Could you check a few things on this model? Use its own coordinates, in mm. A direction names the side the tool comes from. Round coordinates to 2 decimals unless told otherwise and drop trailing zeros. Write each loop counter-clockwise with the first axis right and the second up, starting at its lowest first coordinate (ties: lowest second). Pieces come first, ordered by that corner, then holes. Notation, with made-up numbers: M 20,42 L 28,42 A11 ccw 28,60 Z; hole C 54.5,69.25 d8. An arc over 180 degrees is marked long. One line per item, written item: value. Start each with the question number.
(1) I want a section at C-C on z = 0.85. Count the separate pieces of the cut face and the enclosed holes in it, and give its area (3 significant figures).
(2) I want a section at B-B on y = 25. Please give me the cut outline in (x, z).
(3) Which directions (+Z, -Z, +X, -X, +Y, -Y) give clear straight access to the entire face, cutting with the end or side of a thin tool? Please do faces 4 (the face through (-35, 50.619, 2)), 5 (the face through (-23, 19.156, 2)), 6 (the face through (-1, 37.156, 2)), 7 (the face through (-14.653, 5, 2)).
(4) I want a section at A-A on x = -29.5. Please give me the cut outline in (y, z), and give its area (3 significant figures).
(5) I'm going to push flat-ended pins straight in: pin 1 Ø2 at (x, z) = (0, 1) entering from -Y; pin 2 Ø2 at (x, z) = (-44.5, 3) entering from -Y; pin 3 Ø3 at (x, y) = (-20.38, 14.02) entering from +Z; pin 4 Ø2 at (x, z) = (-1, 2.5) entering from +Y. Where does each tip first touch, or does it pass through?
(6) If I drill on L1, parallel to X at y = 39.5, z = 3.7; L2, parallel to X at y = 34.5, z = 3.85; L3, parallel to X at y = 44, z = 1.3, over which ranges is the centre line in solid material (lowest first)?
(7) Thinking about a two-plate mould opening in Y: for faces 1 (the face through (-11, 37.156, 2)), 2 (the face through (2.101, 15, 2)), 3 (the face through (0.6, 4.99, 1.97)), which applies, released by +Y, released by -Y, zero draft, split by the parting line, or undercut?
```python
from build123d import *

# Parameters (mm, degrees)
SKETCH1_R           = 1.55
BOSS_EXTRUDE1_DEPTH = 4
SKETCH2_R           = 11.25
CUT_EXTRUDE1_DEPTH  = 10
SKETCH4_R           = 2
SKETCH4_W           = 16.7545444
SKETCH4_H           = 7.593360653
BOSS_EXTRUDE2_DEPTH = 4
SKETCH5_R           = 2.001806379
CUT_EXTRUDE2_DEPTH  = 79.038052705
FILLET1_R           = 5


with BuildPart() as part:
    # Sketch1 → Boss-Extrude1 (new body)
    with BuildSketch(Plane.XY):
        Polygon((-6.898627884, 24.176481231), (-6.898627884, 21.876481231), (-14.898627884, 21.876481231), (-14.898627884, 19.156481231), (-46.856968571, 19.156481231), (-46.856968571, 39.876481231), (-14.898627884, 39.876481231), (-14.898627884, 37.156481231), (-6.898627884, 37.156481231), (-6.898627884, 34.856481231), (-7.878627884, 34.856481231), (-7.878627884, 32.800088029), (-7.031414289, 32.376481231), (-3.77584148, 32.376481231), (-2.928627884, 32.800088029), (-2.928627884, 34.856481231), (-3.898627884, 34.856481231), (-3.898627884, 37.156481231), (2.101372116, 37.156481231), (2.101372116, 47.876481231), (2.101372116, 50.619437371), (-56.558762416, 50.619437371), (-56.558762416, 47.876481231), (-56.558762416, 39.876481231), (-56.558762416, 19.156481231), (-56.558762416, 11.156481231), (2.101372116, 11.156481231), (2.101372116, 21.876481231), (-3.898627884, 21.876481231), (-3.898627884, 24.176481231), (-2.928627884, 24.176481231), (-2.928627884, 26.232874433), (-3.77584148, 26.656481231), (-7.031414289, 26.656481231), (-7.878627884, 26.232874433), (-7.878627884, 24.176481231), align=None)
        with Locations((-51.378627884, 14.016481231)):
            Circle(SKETCH1_R, mode=Mode.SUBTRACT)
        with Locations((-20.378627884, 14.016481231)):
            Circle(SKETCH1_R, mode=Mode.SUBTRACT)
        with Locations((-51.378627884, 45.016481231)):
            Circle(SKETCH1_R, mode=Mode.SUBTRACT)
        with Locations((-20.378627884, 45.016481231)):
            Circle(SKETCH1_R, mode=Mode.SUBTRACT)
    extrude(amount=BOSS_EXTRUDE1_DEPTH)

    # Sketch2 → Cut-Extrude1 (cut)
    with BuildSketch(Plane.XY.offset(4)):
        with Locations((-35.878627884, 29.516481231)):
            Circle(SKETCH2_R)
    extrude(amount=-CUT_EXTRUDE1_DEPTH, mode=Mode.SUBTRACT)

    # Sketch4 → Boss-Extrude2 (add)
    # profile 1 of 2: a face of its own
    with BuildSketch(Plane(origin=(0, 0, 0), x_dir=(-1, 0, 0), z_dir=(0, 0, -1))):
        Polygon((-2.101372116, 50.619437371), (-2.101372116, 53.619437371), (15.109222475, 53.619437371), (15.109222475, 50.619437371), (15.109222475, 46.213030652), (-2.101372116, 46.03430596), align=None)
        with Locations((5.403627884, 49.175308869)):
            Circle(SKETCH4_R, mode=Mode.SUBTRACT)
    # profile 2 of 2: a face of its own
    with BuildSketch(Plane(origin=(0, 0, 0), x_dir=(-1, 0, 0), z_dir=(0, 0, -1))):
        with Locations((6.275900084, 7.359800905)):
            Rectangle(SKETCH4_W, SKETCH4_H)
        with Locations((5.403627884, 7.956481231)):
            Circle(SKETCH4_R, mode=Mode.SUBTRACT)
    extrude(amount=-BOSS_EXTRUDE2_DEPTH)

    # Sketch5 → Cut-Extrude2 (cut, through all)
    with BuildSketch(Plane(origin=(0, 0, 0), x_dir=(-1, 0, 0), z_dir=(0, 0, -1))):
        with Locations((5.440315917, 49.166162951)):
            Circle(SKETCH5_R)
    extrude(amount=-CUT_EXTRUDE2_DEPTH, mode=Mode.SUBTRACT)

    # Fillet1
    # the kernel refuses this fillet: 5 mm, written as the material it adds along each edge
    with BuildSketch(Plane(origin=(-14.653172284, 11.156481231, 0), x_dir=(0, -1, 0), z_dir=(0, 0, 1))) as fillet1_piece_1:
        with BuildLine():
            CenterArc((FILLET1_R, -FILLET1_R), FILLET1_R, 90, 90)
            Line((0, -FILLET1_R), (0, 0))
            Line((0, 0), (FILLET1_R, 0))
        make_face()
    extrude(amount=4)
    with BuildSketch(Plane(origin=(-15.109222475, 50.619437371, 0), x_dir=(-1, 0, 0), z_dir=(0, 0, 1))) as fillet1_piece_2:
        with BuildLine():
            CenterArc((4.582575695, -5), FILLET1_R, 90, 66.421821522)
            Line((0, -3), (0, 0))
            Line((0, 0), (4.582575695, 0))
        make_face()
    extrude(amount=4)
    # the kernel refuses this fillet: 5 mm, written as the material it takes off along each edge
    with BuildSketch(Plane(origin=(2.101372116, 53.619437371, -12.5), x_dir=(0, -1, 0), z_dir=(0, 0, 1)), Plane(origin=(2.101372116, 3.563120578, -12.5), x_dir=(-1, 0, 0), z_dir=(0, 0, 1)), Plane(origin=(-56.558762416, 11.156481231, -12.5), x_dir=(0, 1, 0), z_dir=(0, 0, 1)), Plane(origin=(-56.558762416, 50.619437371, -12.5), x_dir=(1, 0, 0), z_dir=(0, 0, 1))) as fillet1_2_piece_1:
        with BuildLine():
            CenterArc((FILLET1_R, -FILLET1_R), FILLET1_R, 90, 90)
            Line((0, -FILLET1_R), (0, 0))
            Line((0, 0), (FILLET1_R, 0))
        make_face()
    extrude(amount=29, mode=Mode.SUBTRACT)


solid = part.part
```
Found:
1. separate pieces: 1
1. enclosed holes: 6
1. area: 1,530 mm²
2. outline: M -56.56,0 L -46.86,0 L -46.86,4 L -56.56,4 Z; M -7.88,0 L -2.93,0 L -2.93,4 L -7.88,4 Z
3. face 4: +Z, -Z, -X, +Y
3. face 5: +Z, -Z
3. face 6: +Z, -Z, +X
3. face 7: +Z, -Z, -X, -Y
4. outline: M 11.16,0 L 19.16,0 L 19.16,4 L 11.16,4 Z; M 39.88,0 L 50.62,0 L 50.62,4 L 39.88,4 Z
4. area: 75.0 mm²
5. pin 1: stops at y = 3.94
5. pin 2: stops at y = 11.16
5. pin 3: passes through
5. pin 4: stops at y = 53.54
6. L1: x = -56.56 to -46.86, -14.9 to 2.1
6. L2: x = -56.56 to -46.86, -7.88 to -2.93
6. L3: x = -56.56 to -52.55, -50.21 to -21.55, -19.21 to 2.1
7. face 1: undercut
7. face 2: zero draft
7. face 3: released by -Y
